Can you work these out from the model? Positions are in its coordinate system, mm. A direction names the side the tool comes from. Coordinates: 2 decimals unless noted, no trailing zeros. Order: outer loops, then holes, each group sorted by start corner. A loop starts at its lowest first (then second) coordinate and runs counter-clockwise, first axis right, second up. Notation, with made-up numbers: (43, 79.5) -> (64, 79.5) arc R24 ccw to (64, 106.5) -> close; hole circle Ø1 at (55, 56.25). An arc over 180 degrees is marked (long way). Use a Markdown table: item, result. Add a question column.
1. We'd pull the mould along Y, two halves only. Please class faces 4 (the flat face through (-0.36, 5.73, -3.07)), 5 (the flat face through (0, 52, 1)), 6 (the flat face through (0, 51.3, 1)): pulls with the +Y half, pulls with the -Y half, needs draft (parallel to the pull), parting line crosses it, or undercut.
2. Suppose I cut it at A-A, the plane x = 0. List the corners of the cut face in (y, z) for me, then the cut area to 3 significant figures.
3. Suppose I cut it at C-C, the plane y = 42. List the corners of the cut face in (x, z) for me, then the cut area to 3 significant figures.
4. For pin 1 Ø8 at (x, y) = (5, 15.5) entering from -Z; pin 2 Ø1 at (x, y) = (19, 25) entering from -Z; pin 3 Ø1.5 at (x, y) = (-5.5, 19.5) entering from -Z, each with a flat end and sliding along its axis, tell me the tip position at first contact or that it passes through.
5. Suppose I cut it at B-B, the plane y = 8.5. List the corners of the cut face in (x, z) for me, then the cut area to 3 significant figures.
6. For faces 1 (the cylindrical face through (-0.556, 28.109, 12.294)), 2 (the cylindrical face through (-0.572, 27.789, 12.994)), 3 (the cylindrical face through (-0.264, 51.655, -1.003)), which set-ups out of +Z, -Z, +X, -X, +Y, -Y let a thin tool reach every point of the face, with its end or its side?
7. If I drill on line 1 along Y through (x, z) = (14, 5); line 2 along X through (y, z) = (48, 3); line 3 along Y through (x, z) = (-19.5, -8.5), over which ranges is the centre line in solid material (lowest first)? Write a range as from..to.
```python
from build123d import *

# Parameters (mm, degrees)
BOSS_EXTRUDE1_DEPTH     = 52
FILLET1_R               = 6
CUT_EXTRUDE1_DEPTH      = 60.573484078
CUT_EXTRUDE1_DEPTH_BACK = 60.573484078
SHELL1_T                = -0.7
SKETCH3_R               = 12
CUT_EXTRUDE2_DEPTH      = 32


with BuildPart() as part:
    # Sketch1 → Boss-Extrude1 (new body)
    with BuildSketch(Plane(origin=(0, 0, 0), x_dir=(1, 0, 0), z_dir=(0, 1, 0))):
        with BuildLine():
            Line((26, 13), (-26, 13))
            ThreePointArc((-26, 13), (0, -13), (26, 13))
        make_face()
    extrude(amount=BOSS_EXTRUDE1_DEPTH)

    # Fillet1
    fillet1_edges = [part.edges().sort_by_distance(p)[0] for p in [
        (0, 52, 13),
    ]]
    fillet(fillet1_edges, radius=FILLET1_R)

    # Sketch2 → Cut-Extrude1 (cut, two sides: drawn at the far end of the back side and taken through both)
    with BuildSketch(Plane(origin=(0, 0, 0), x_dir=(0, 0, -1), z_dir=(1, 0, 0)).offset(-CUT_EXTRUDE1_DEPTH_BACK)):
        Polygon((13, 0), (-13, 15), (-13, 0), align=None)
    extrude(amount=CUT_EXTRUDE1_DEPTH + CUT_EXTRUDE1_DEPTH_BACK, mode=Mode.SUBTRACT)

    # Shell1
    shell1_openings = [part.faces().sort_by_distance(p)[0] for p in [
        (0, 25.858277944, -13),
    ]]
    offset(amount=SHELL1_T, openings=shell1_openings)

    # Sketch3 → Cut-Extrude2 (cut)
    with BuildSketch(Plane(origin=(0, 52, 0), x_dir=(1, 0, 0), z_dir=(0, 1, 0))):
        with Locations((0, 13)):
            Circle(SKETCH3_R)
    extrude(amount=-CUT_EXTRUDE2_DEPTH, mode=Mode.SUBTRACT)


solid = part.part
```
Worked out:
| question | item | result |
|---|---|---|
| 1 | face 4 | pulls with the -Y half |
| 1 | face 5 | pulls with the +Y half |
| 1 | face 6 | undercut |
| 2 | outline | (0, -13) -> (0.81, -13) -> (15.4, 12.3) -> (46, 12.3) arc R5.3 cw to (51.3, 7) -> (51.3, -1) -> (52, -1) -> (52, 7) arc R6 ccw to (46, 13) -> (15, 13) -> close |
| 2 | area | 54.1 mm² |
| 3 | outline | (-26, -13) -> (-25.3, -13) arc R25.3 cw to (25.3, -13) -> (26, -13) arc R26 ccw to start |
| 3 | area | 56.4 mm² |
| 4 | pin 1 | stops at z = 5.53 |
| 4 | pin 2 | stops at z = 3.12 |
| 4 | pin 3 | stops at z = 11.52 |
| 5 | outline | (-26, -13) -> (-25.3, -13) arc R25.3 cw to (-21.5, 0.33) -> (21.5, 0.33) arc R25.3 cw to (25.3, -13) -> (26, -13) arc R26 ccw to (21.42, 1.73) -> (-21.42, 1.73) arc R26 ccw to start |
| 5 | area | 80.9 mm² |
| 6 | face 1 | -Z |
| 6 | face 2 | +Z, +Y, -Y |
| 6 | face 3 | -Z, +Y |
| 7 | line 1 | y = 10.38..11.19, 50.5..51.3 |
| 7 | line 2 | x = -20.06..-19.09, 19.09..20.06 |
| 7 | line 3 | y = 2.6..3.4, 51.3..52 |
